Check sheet for the modelled part. Datum: model origin and axes. Units: mm. Round coordinates to 2 decimals unless told otherwise and drop trailing zeros. Order: outer loops, then holes, each group sorted by start corner. A loop starts at its lowest first (then second) coordinate and runs counter-clockwise, first axis right, second up. Notation, with made-up numbers: (37.25, 7) -> (62.25, 7) arc R14 cw to (62.25, 23) -> close; hole circle Ø9 at (8.25, 85). An arc over 180 degrees is marked (long way). Answer in a Markdown table with one row per item.
Autodesk Inventor part; units mm, degrees
ref_plane "YZ Plane" through (0, 0, 0) normal (1, 0, 0) x (0, 1, 0)
ref_plane "XZ Plane" through (0, 0, 0) normal (0, 1, 0) x (-1, 0, 0)
ref_plane "XY Plane" through (0, 0, 0) normal (0, 0, 1) x (1, 0, 0)
sketch "Sketch1" plane through (0, 0, 0) normal (0, 1, 0) x (-1, 0, 0)
  circle A0 centre (0, 0) radius 115
  circle A1 centre (0, 0) radius 16
  dimension "d0" = 230
  dimension "d1" = 32
extrude "Extrusion1" add sketch "Sketch1" along normal blind 6.35
sketch "Sketch2" plane through (0, 6.35, 0) normal (0, 1, 0) x (1, 0, 0)
  circle A0 centre (0, 56) radius 4
  circle A1 centre (-28, 48.4974) radius 4
  circle A2 centre (-48.4974, 28) radius 4
  circle A3 centre (-56, 0) radius 4
  circle A4 centre (-48.4974, -28) radius 4
  circle A5 centre (-28, -48.4974) radius 4
  circle A6 centre (0, -56) radius 4
  circle A7 centre (28, -48.4974) radius 4
  circle A8 centre (48.4974, -28) radius 4
  circle A9 centre (56, 0) radius 4
  circle A10 centre (48.4974, 28) radius 4
  circle A11 centre (28, 48.4974) radius 4
  point P0 (0, 0)
  dimension "d4" = 8
  dimension "d5" = 56
  dimension "d8" = 360
extrude "Extrusion2" cut sketch "Sketch2" against normal through all
sketch "Sketch4" plane through (0, 6.35, 0) normal (0, 1, 0) x (1, 0, 0)
  circle A0 centre (-36, 84) radius 7
  circle A1 centre (-44, 100) radius 2
  line L0 (-36, 91) -> (-36, 77) construction
  line L1 (-43, 84) -> (-29, 84) construction
  circle A2 centre (-28, 100) radius 2
  circle A3 centre (-44, 68) radius 2
  circle A4 centre (-28, 68) radius 2
  circle A5 centre (0, 0) radius 16 construction
  line L2 (0, 16) -> (0, -16) construction
  line L3 (-16, 0) -> (16, 0) construction
  circle A6 centre (36, 84) radius 7
  circle A7 centre (44, 100) radius 2
  circle A8 centre (28, 100) radius 2
  circle A9 centre (44, 68) radius 2
  circle A10 centre (28, 68) radius 2
  circle A11 centre (-36, -84) radius 7
  circle A12 centre (-44, -100) radius 2
  circle A13 centre (-28, -100) radius 2
  circle A14 centre (-44, -68) radius 2
  circle A15 centre (-28, -68) radius 2
  circle A16 centre (36, -84) radius 7
  circle A17 centre (44, -100) radius 2
  circle A18 centre (28, -100) radius 2
  circle A19 centre (28, -68) radius 2
  circle A20 centre (44, -68) radius 2
  circle A21 centre (0, 0) radius 64 construction
  point P0 (-29, -84)
  dimension "d34" = 14
  dimension "d35" = 36
  dimension "d36" = 84
  dimension "d37" = 4
  dimension "d38" = 8
  dimension "d39" = 16
  dimension "d42" = 128
extrude "Extrusion4" cut sketch "Sketch4" against normal through all
properties part number "ArmBase"
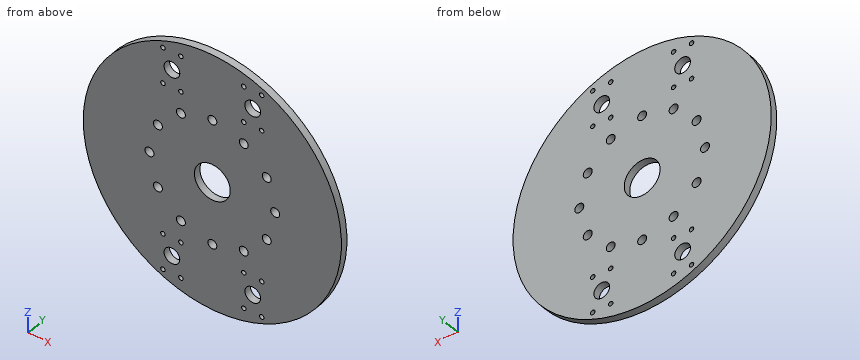
Item 1: Scan lines: line 1 (Z direction, x = 0, y = 3.75); line 2 (Z direction, x = 36, y = 5); line 3 (Z direction, x = 37, y = 0.5). Record each from-to range of solid material in increasing order. Write a range as [from, to].
Result sheet:
| item | result |
|---|---|
| line 1 | z = [-115, -60], [-52, -16], [16, 52], [60, 115] |
| line 2 | z = [-109.22, -91], [-77, 77], [91, 109.22] |
| line 3 | z = [-108.89, -90.93], [-77.07, 77.07], [90.93, 108.89] |
Item 2: Cross-section at C-C (z = -84). Record the boundary of the cut face in (x, y), and give its area (3 significant figures).
Result sheet:
| item | result |
|---|---|
| outline | (-78.54, 0) -> (-43, 0) -> (-43, 6.35) -> (-78.54, 6.35) -> close; (-29, 0) -> (29, 0) -> (29, 6.35) -> (-29, 6.35) -> close; (43, 0) -> (78.54, 0) -> (78.54, 6.35) -> (43, 6.35) -> close |
| area | 820 mm^2 |
Item 3: Cross-section at B-B (x = 49). Record the boundary of the cut face in (y, z), and give its area (3 significant figures).
Result sheet:
| item | result |
|---|---|
| outline | (0, -104.04) -> (6.35, -104.04) -> (6.35, -31.97) -> (0, -31.97) -> close; (0, -24.03) -> (6.35, -24.03) -> (6.35, 24.03) -> (0, 24.03) -> close; (0, 31.97) -> (6.35, 31.97) -> (6.35, 104.04) -> (0, 104.04) -> close |
| area | 1,220 mm^2 |
Item 4: Cross-section at D-D (x = -56). Record the boundary of the cut face in (y, z), and give its area (3 significant figures).
Result sheet:
| item | result |
|---|---|
| outline | (0, -100.44) -> (6.35, -100.44) -> (6.35, -4) -> (0, -4) -> close; (0, 4) -> (6.35, 4) -> (6.35, 100.44) -> (0, 100.44) -> close |
| area | 1,220 mm^2 |
Item 5: Depth check by flat-ended pin: P1, Ø5, axis at x = 28, z = -68, coming from the +Y side; P2, Ø2, axis at x = 82.5, y = 2, coming from the +Z side; P3, Ø1, axis at x = -38, y = 4, coming from the -Z side; P4, Ø1.5, axis at x = -73.5, y = 3.5, coming from the +Z side. Enter the tip coordinate at first touch or a pass-through.
Result sheet:
| item | result |
|---|---|
| P1 | stops at y = 6.35 |
| P2 | stops at z = 81.13 |
| P3 | stops at z = -108.71 |
| P4 | stops at z = 89.06 |
Item 6: Cross-section at A-A (z = 0). Record the boundary of the cut face in (x, y), and give its area (3 significant figures).
Result sheet:
| item | result |
|---|---|
| outline | (-115, 0) -> (-60, 0) -> (-60, 6.35) -> (-115, 6.35) -> close; (-52, 0) -> (-16, 0) -> (-16, 6.35) -> (-52, 6.35) -> close; (16, 0) -> (52, 0) -> (52, 6.35) -> (16, 6.35) -> close; (60, 0) -> (115, 0) -> (115, 6.35) -> (60, 6.35) -> close |
| area | 1,160 mm^2 |
